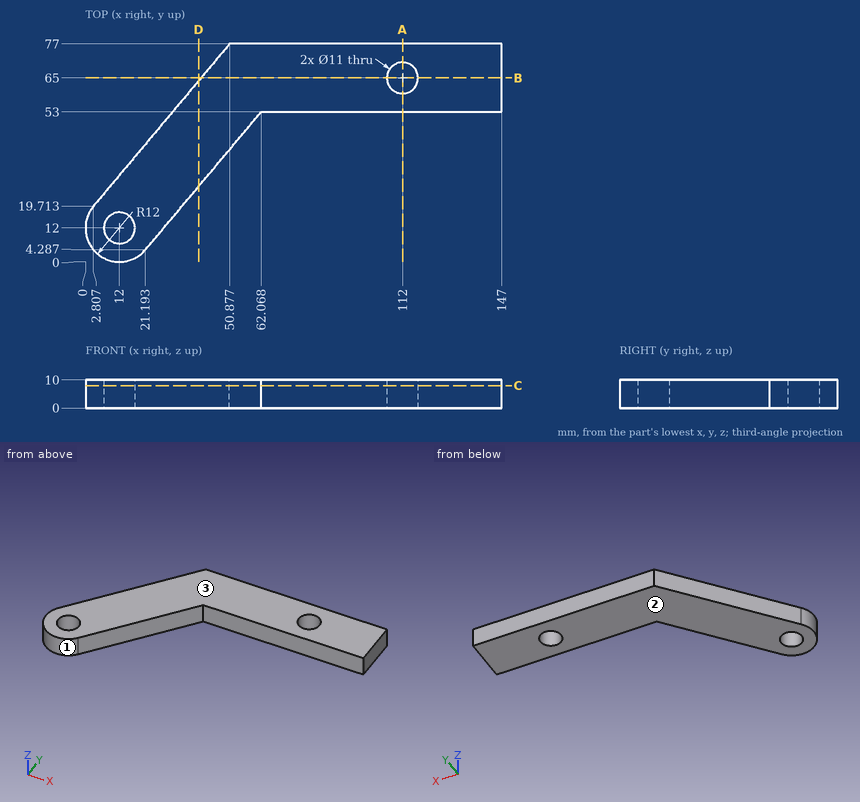
Geometry: see drawing. Coordinates: mm, zero at the bounding-box minimum. Coordinates: 2 decimals unless noted, no trailing zeros. Loops run counter-clockwise (first coordinate to the right, second up) from the corner with the lowest first, then second, coordinate; pieces in that order, holes last. Notation, with made-up numbers: (45.25, 8.25) - (66.25, 8.25) arc R27 ccw to (66.25, 43.25) - close; hole circle Ø11 at (74, -18). An arc over 180 degrees is marked (long way). Return JSON: item names as keys, results as strings.
Q1. Contact query for flat-ended pins moving along their axis: P1, Ø5, axis at x = 66, z = 5.5, coming from the -Y side; P2, Ø6.5, axis at x = 12, y = 12, coming from the -Z side; P3, Ø4, axis at x = 27, z = 3.5, coming from the -Y side (1 decimal). Output: stop coordinate, or through.
Results:
{"P1": "y = 53", "P2": "through", "P3": "y = 8.8"}
Q2. Section B-B, the plane y = 65. Return loops of the section in (x, z), plus the area to 3 significant figures.
Results:
{"outline": "(40.81, 0) - (106.5, 0) - (106.5, 10) - (40.81, 10) - close; (117.5, 0) - (147, 0) - (147, 10) - (117.5, 10) - close", "area": "952 mm2"}
Q3. Section A-A, the plane x = 112. Return loops of the section in (y, z).
Results:
{"outline": "(53, 0) - (59.5, 0) - (59.5, 10) - (53, 10) - close; (70.5, 0) - (77, 0) - (77, 10) - (70.5, 10) - close"}
Q4. Section D-D, the plane x = 40. Return loops of the section in (y, z), plus the area to 3 significant figures.
Results:
{"outline": "(26.7, 0) - (64.04, 0) - (64.04, 10) - (26.7, 10) - close", "area": "373 mm2"}
Q5. Mould query, pull axis Z, two halves, no side actions, for the marked faces 1, 2 and 3. Classes: released by +Z, released by -Z, zero draft, split by the parting line, or undercut.
Results:
{"face 1": "zero draft", "face 2": "released by -Z", "face 3": "released by +Z"}
Q6. Material intervals for line 1 along Y through (x, z) = (112, 6); line 2 along X through (y, z) = (17, 6.25) (1 decimal); line 3 along X through (y, z) = (12, 6) (1 decimal), sorted ascending.
Results:
{"line 1": "53 to 59.5, 70.5 to 77", "line 2": "1.1 to 9.7, 14.3 to 31.9", "line 3": "0 to 6.5, 17.5 to 27.7"}
Q7. Section C-C, the plane z = 8. Return loops of the section in (x, y), plus the area to 3 significant figures.
Results:
{"outline": "(2.81, 19.71) arc R12 ccw to (21.19, 4.29) - (62.07, 53) - (147, 53) - (147, 77) - (50.88, 77) - close; hole circle Ø11 at (12, 12); hole circle Ø11 at (112, 65)", "area": "3,870 mm2"}
